Geometry check sheet. Reference: the model listing, model coordinates, mm. Give positions to 0.01 mm unless a question says otherwise; leave off trailing zeros. Write each loop counter-clockwise with the first axis right and the second up, starting at its lowest first coordinate (ties: lowest second). Pieces come first, ordered by that corner, then holes. Notation, with made-up numbers: (32.5, -37) - (63.5, -37) arc R28 cw to (63.5, -1) - close; hole circle Ø7 at (-27.5, 78). An arc over 180 degrees is marked (long way). One line per question, with ' | ' between items. Start each with the question number.
Q1. Thickness scan on L1, parallel to Y at x = 138, z = 2 (3 decimals); L2, parallel to Y at x = -69, z = 3 (3 decimals); L3, parallel to X at y = 12.5, z = 0.5. Record the ranges inside material, lowest first. Write a range as [from, to].
Q2. Section check C-C on z = 3. Count the separate pieces of the cut face and the enclosed holes in it, and give its area (3 significant figures).
Q3. Release check for a two-part mould opening along X. For faces 1 (the face through (81.232, 0.474, 3.131)), 2 (the face through (-152.4, 0, 3)), 3 (the face through (-2, 11, 0)) record: +X half, -X half, draft (parallel to the pull), parting line (faces both ways), or undercut.
Q4. Section check A-A on x = 92. Record the boundary of the cut face in (y, z) (3 decimals), and give its area (3 significant figures).
Q5. Section check B-B on x = -23. Record the boundary of the cut face in (y, z) (3 decimals).
Q6. Gauge pin test, flat end, axial feed: P1, Ø5, axis at x = -79, y = 8.5, coming from the -Z side. Record the tip position at first contact, or that the pin passes through.
```python
from build123d import *

# Parameters (mm, degrees)
SKETCH1_W           = 304.8
SKETCH1_H           = 31.75
SKETCH1_R           = 10.575
SKETCH1_R_2         = 10.6258
SKETCH1_R_3         = 10.6766
SKETCH1_R_4         = 10.7274
SKETCH1_R_5         = 10.7782
SKETCH1_R_6         = 10.829
SKETCH1_R_7         = 10.8798
SKETCH1_R_8         = 10.2702
SKETCH1_R_9         = 10.321
SKETCH1_R_10        = 10.3718
SKETCH1_R_11        = 10.4226
SKETCH1_R_12        = 10.4734
SKETCH1_R_13        = 10.5242
SKETCH1_R_14        = 1.5
BOSS_EXTRUDE1_DEPTH = 6.35


with BuildPart() as part:
    # Sketch1 → Boss-Extrude1 (new body)
    with BuildSketch(Plane.XY):
        Rectangle(SKETCH1_W, SKETCH1_H)
        Circle(SKETCH1_R, mode=Mode.SUBTRACT)
        with Locations((23, 0)):
            Circle(SKETCH1_R_2, mode=Mode.SUBTRACT)
        with Locations((46, 0)):
            Circle(SKETCH1_R_3, mode=Mode.SUBTRACT)
        with Locations((69, 0)):
            Circle(SKETCH1_R_4, mode=Mode.SUBTRACT)
        with Locations((92, 0)):
            Circle(SKETCH1_R_5, mode=Mode.SUBTRACT)
        with Locations((115, 0)):
            Circle(SKETCH1_R_6, mode=Mode.SUBTRACT)
        with Locations((138, 0)):
            Circle(SKETCH1_R_7, mode=Mode.SUBTRACT)
        with Locations(Location((-138, 0, 0), (0, 0, 180))):
            Circle(SKETCH1_R_8, mode=Mode.SUBTRACT)
        with Locations(Location((-115, 0, 0), (0, 0, 180))):
            Circle(SKETCH1_R_9, mode=Mode.SUBTRACT)
        with Locations(Location((-92, 0, 0), (0, 0, 180))):
            Circle(SKETCH1_R_10, mode=Mode.SUBTRACT)
        with Locations(Location((-69, 0, 0), (0, 0, 180))):
            Circle(SKETCH1_R_11, mode=Mode.SUBTRACT)
        with Locations(Location((-46, 0, 0), (0, 0, 180))):
            Circle(SKETCH1_R_12, mode=Mode.SUBTRACT)
        with Locations(Location((-23, 0, 0), (0, 0, 180))):
            Circle(SKETCH1_R_13, mode=Mode.SUBTRACT)
        with Locations((148.807897552, 12.282897552)):
            Circle(SKETCH1_R_14, mode=Mode.SUBTRACT)
    extrude(amount=BOSS_EXTRUDE1_DEPTH)


solid = part.part
```
Working result:
1) L1: y = [-15.875, -10.88], [10.88, 15.875] | L2: y = [-15.875, -10.423], [10.423, 15.875] | L3: x = [-152.4, 147.32], [150.29, 152.4]
2) separate pieces: 1 | enclosed holes: 14 | area: 5,100 mm2
3) face 1: undercut | face 2: -X half | face 3: draft
4) outline: (-15.875, 0) - (-10.778, 0) - (-10.778, 6.35) - (-15.875, 6.35) - close; (10.778, 0) - (15.875, 0) - (15.875, 6.35) - (10.778, 6.35) - close | area: 64.7 mm2
5) outline: (-15.875, 0) - (-10.524, 0) - (-10.524, 6.35) - (-15.875, 6.35) - close; (10.524, 0) - (15.875, 0) - (15.875, 6.35) - (10.524, 6.35) - close
6) P1: stops at z = 0
